from build123d import *

# Parameters (mm, degrees)
CROQUIS1_W              = 70
CROQUIS1_H              = 50
SALIENTE_EXTRUIR1_DEPTH = 50
CROQUIS2_W              = 50
CROQUIS2_H              = 50
SALIENTE_EXTRUIR2_DEPTH = 180
CROQUIS3_W              = 40
CROQUIS3_H              = 40
CORTAR_EXTRUIR1_DEPTH   = 170
CORTAR_EXTRUIR2_DEPTH   = 50


with BuildPart() as part:
    # Croquis1 → Saliente-Extruir1 (new body)
    with BuildSketch(Plane.XY):
        Rectangle(CROQUIS1_W, CROQUIS1_H)
    extrude(amount=SALIENTE_EXTRUIR1_DEPTH)

    # Croquis2 → Saliente-Extruir2 (add)
    with BuildSketch(Plane.ZY.offset(35)):
        with Locations((75, 0)):
            Rectangle(CROQUIS2_W, CROQUIS2_H)
    extrude(amount=-SALIENTE_EXTRUIR2_DEPTH)

    # Croquis3 → Cortar-Extruir1 (cut)
    with BuildSketch(Plane(origin=(145, 0, 0), x_dir=(0, 0, -1), z_dir=(1, 0, 0))):
        with Locations((-75, 0)):
            Rectangle(CROQUIS3_W, CROQUIS3_H)
    extrude(amount=-CORTAR_EXTRUIR1_DEPTH, mode=Mode.SUBTRACT)

    # Croquis4 → Cortar-Extruir2 (cut)
    with BuildSketch(Plane.XZ.offset(25)):
        Polygon((60, 85), (-25, 85), (-25, 65), (60, 65), (130, 65), (130, 85), align=None)
    extrude(amount=-CORTAR_EXTRUIR2_DEPTH, mode=Mode.SUBTRACT)


solid = part.part
CAD build for the part. Positions are in the model's coordinates, mm. A direction names the side the tool comes from. Round coordinates to 2 decimals unless told otherwise and drop trailing zeros. Write each loop counter-clockwise with the first axis right and the second up, starting at its lowest first coordinate (ties: lowest second). Pieces come first, ordered by that corner, then holes. Notation, with made-up numbers: (78.25, 40.25) -> (87.25, 40.25) arc R28 cw to (87.25, 62.25) -> close; hole circle Ø5 at (69, -26.75). An arc over 180 degrees is marked (long way). Answer as a JSON object with one key per item and string values.
(1) Band-saw the part on D-D, the plane y = 7. List the corners of the cut face in (x, z).
Reported:
{"outline": "(-35, 0) -> (35, 0) -> (35, 50) -> (145, 50) -> (145, 55) -> (-25, 55) -> (-25, 95) -> (145, 95) -> (145, 100) -> (-35, 100) -> close"}
(2) Pin check, flat tips, straight feed: P1, Ø15, axis at x = 79, y = -9.5, coming from the -Z side; P2, Ø1.5, axis at y = 11, z = 35.5, coming from the +X side; P3, Ø12, axis at y = -1.5, z = 65.5, coming from the +X side. Stop position of each tip, or through.
Reported:
{"P1": "stops at z = 50", "P2": "stops at x = 35", "P3": "stops at x = -25"}
(3) Two-plate mould, pull along Y, no slides. Class faces 4 (the face through (34, -25, 49)), 5 (the face through (61, 0, 95)), 6 (the face through (89, 0, 50)): +Y half, -Y half, draft (parallel to the pull), parting line (faces both ways), or undercut.
Reported:
{"face 4": "-Y half", "face 5": "undercut", "face 6": "draft"}
(4) Band-saw the part on C-C, the plane z = 57.5. List the corners of the cut face in (x, y).
Reported:
{"outline": "(-35, -25) -> (145, -25) -> (145, -20) -> (-25, -20) -> (-25, 20) -> (145, 20) -> (145, 25) -> (-35, 25) -> close"}
(5) Band-saw the part on A-A, the plane x = -2. List the corners of the cut face in (y, z).
Reported:
{"outline": "(-25, 0) -> (25, 0) -> (25, 65) -> (20, 65) -> (20, 55) -> (-20, 55) -> (-20, 65) -> (-25, 65) -> close; (-25, 85) -> (-20, 85) -> (-20, 95) -> (20, 95) -> (20, 85) -> (25, 85) -> (25, 100) -> (-25, 100) -> close"}
(6) Probe probe 1 along Z at (x, y) = (17.5, 0); probe 2 along Y at (x, z) = (10, 59); probe 3 along Z at (x, y) = (103, -7). List the from-to ranges inside material, lowest first. Write a range as [from, to].
Reported:
{"probe 1": "z = [0, 55], [95, 100]", "probe 2": "y = [-25, -20], [20, 25]", "probe 3": "z = [50, 55], [95, 100]"}
(7) Which spindle directions (+Z, -Z, +X, -X, +Y, -Y) get a long thin tool onto all of the face, cutting with end or side? Do faces 1 (the face through (35, 0, 25)), 2 (the face through (130, 22, 75)), 3 (the face through (61, 20, 89)). Say none if no direction does.
Reported:
{"face 1": "-Z, +X, +Y, -Y", "face 2": "+Y, -Y", "face 3": "+X"}
(8) Band-saw the part on B-B, the plane z = 74. List the corners of the cut face in (x, y).
Reported:
{"outline": "(-35, -25) -> (-25, -25) -> (-25, 25) -> (-35, 25) -> close; (130, -25) -> (145, -25) -> (145, -20) -> (130, -20) -> close; (130, 20) -> (145, 20) -> (145, 25) -> (130, 25) -> close"}
